```python
from build123d import *

# Parameters (mm, degrees)
F1_DEPTH = 70
F3_DEPTH = 70
F4_COUNT = 4
F5_T     = -2
F7_DEPTH = 23
F8_DEPTH = 2


with BuildPart() as f1:
    # F0 (on Front) → F1 (new body)
    with BuildSketch(Plane.XZ):
        Polygon((0, 25), (0, 0), (68, 0), (68, 2), (70, 4), (70, 25), align=None)
    extrude(amount=-F1_DEPTH)

    # F2 (on Right) → F3 (intersect, through all)
    with BuildSketch(Plane.YZ):
        Polygon((0, 25), (0, 0), (68, 0), (68, 2), (70, 4), (70, 25), align=None)
    extrude(amount=F3_DEPTH, mode=Mode.INTERSECT)

    # F4: F1 ×4 about axis
    f4_axis = Axis((0, 0, 12.5), (0, 0, 1))


with BuildPart() as f1_1:
    add(f1.part)
    for i in range(1, F4_COUNT):
        add(f1.part.rotate(f4_axis, i * 360 / F4_COUNT))

    # F5
    f5_openings = [f1_1.faces().sort_by_distance(p)[0] for p in [
        (0, 0, 25),
    ]]
    offset(amount=F5_T, openings=f5_openings, kind=Kind.INTERSECTION)

    # F6 (on face) → F7 (join, through all)
    with BuildSketch(Plane.XY.offset(25)):
        Polygon((-66, -66), (-68, -64), (-68, -68), (-64, -68), align=None)
        Polygon((68, -68), (68, -64), (64, -68), align=None)
        Polygon((68, 68), (64, 68), (66, 66), (68, 64), align=None)
        Polygon((-64, 68), (-68, 68), (-68, 64), (-66, 66), align=None)
    extrude(amount=-F7_DEPTH)

    # F6 (on face) → F8 (cut)
    with BuildSketch(Plane.XY.offset(25)):
        Polygon((68, -68), (68, -64), (64, -68), align=None)
        Polygon((68, 68), (64, 68), (66, 66), (68, 64), align=None)
        Polygon((-64, 68), (-68, 68), (-68, 64), (-66, 66), align=None)
        Polygon((-66, -66), (-68, -64), (-68, -68), (-64, -68), align=None)
    extrude(amount=-F8_DEPTH, mode=Mode.SUBTRACT)


solid = f1_1.part
```
The model under review builds one solid part; all positions refer to its coordinate system, in mm. A direction names the side the tool comes from. Give positions to 0.01 mm unless a question says otherwise; leave off trailing zeros. Loops run counter-clockwise (first coordinate to the right, second up) from the corner with the lowest first, then second, coordinate; pieces in that order, holes last. Notation, with made-up numbers: (-15.75, -17) - (19.25, -17) arc R38 ccw to (19.25, 21) - close; hole circle Ø6 at (16.5, 72.5). An arc over 180 degrees is marked (long way). Answer as a JSON object with one key per item and string values.
Q1. Add section B-B on y = 25.5. State the section outline as (x, z) points, plus the area to 3 significant figures.
Worked out:
{"outline": "(-70, 4) - (-68, 2) - (-68, 0) - (68, 0) - (68, 2) - (70, 4) - (70, 25) - (68, 25) - (68, 4.83) - (66, 2.83) - (66, 2) - (-66, 2) - (-66, 2.83) - (-68, 4.83) - (-68, 25) - (-70, 25) - close", "area": "367 mm^2"}
Q2. Insertion check: pin 1 (0.6 mm diameter, centred on y = 18, z = 0.5, fed in from +X); pin 2 (0.7 mm diameter, centred on x = 25.5, z = 2, fed in from -Y); pin 3 (1.6 mm diameter, centred on x = 30.5, z = 0.5, fed in from +Y). Each pin has a flat end and moves straight along its axis. Give the tip position at first contact, or say it passes through.
Worked out:
{"pin 1": "stops at x = 68", "pin 2": "stops at y = -68.35", "pin 3": "stops at y = 68"}
Q3. Add section A-A on z = 9.25. State the section outline as (x, y) points, plus the area to 3 significant figures.
Worked out:
{"outline": "(-70, -70) - (70, -70) - (70, 70) - (-70, 70) - close; hole (-68, -64) - (-64, -68) - (64, -68) - (68, -64) - (68, 64) - (64, 68) - (-64, 68) - (-68, 64) - close", "area": "1,140 mm^2"}
Q4. To check wall thickness, follow line 1 along Y through (x, z) = (14.5, 5); line 2 along Z through (x, y) = (18, -63). State the ranges of each line that lie inside material, in increasing order.
Worked out:
{"line 1": "y = -70 to -68, 68 to 70", "line 2": "z = 0 to 2"}
Q5. For faces 1 (the flat face through (-68, 1, 15)), 2 (the flat face through (-1, 1, 0)), list the 3-axis set-ups (+Z, -Z, +X, -X, +Y, -Y) from which the entire face can be reached by the end or side of a thin tool; tool diameter is ignored.
Worked out:
{"face 1": "+Z", "face 2": "-Z, +X, -X, +Y, -Y"}
Q6. Mouldability with a two-part tool opening along Y and no side actions: class faces 3 (the flat face through (1, 70, 14)), 4 (the flat face through (-1, 1, 2)), 5 (the flat face through (70, 1, 15)) as +Y half, -Y half, draft (parallel to the pull), parting line (faces both ways), or undercut.
Worked out:
{"face 3": "+Y half", "face 4": "undercut", "face 5": "draft"}
